```python
from build123d import *

# Parameters (mm, degrees)
F0_W     = 115
F0_H     = 215
F1_DEPTH = 50
F2_W     = 85
F2_H     = 12
F3_DEPTH = 14
F4_R     = 2
F5_DEPTH = 5
F6_R     = 2
F7_DEPTH = 5


with BuildPart() as f1:
    # F0 (on Front) → F1 (new body)
    with BuildSketch(Plane.XZ):
        with Locations((57.5, 107.5)):
            Rectangle(F0_W, F0_H)
    extrude(amount=F1_DEPTH)

    # F2 (on face) → F3 (join)
    with BuildSketch(Plane.XY.offset(215)):
        with Locations((52.5, -36)):
            Rectangle(F2_W, F2_H)
    extrude(amount=F3_DEPTH)

    # F4 (on face) → F5 (cut)
    with BuildSketch(Plane.XZ.offset(50)):
        with Locations((32.5, 182.5)):
            Circle(F4_R)
        with Locations((82.5, 182.5)):
            Circle(F4_R)
        with Locations((82.5, 32.5)):
            Circle(F4_R)
        with Locations((32.5, 32.5)):
            Circle(F4_R)
    extrude(amount=-F5_DEPTH, mode=Mode.SUBTRACT)

    # F6 (on face) → F7 (cut)
    with BuildSketch(Plane(origin=(0, 0, 0), x_dir=(0, -1, 0), z_dir=(-1, 0, 0))):
        with Locations((12.5, 182.5)):
            Circle(F6_R)
        with Locations((37.5, 182.5)):
            Circle(F6_R)
        with Locations((37.5, 32.5)):
            Circle(F6_R)
        with Locations((12.5, 32.5)):
            Circle(F6_R)
    extrude(amount=-F7_DEPTH, mode=Mode.SUBTRACT)


solid = f1.part
```
Geometry check sheet. Reference: the model listing, model coordinates, mm. A direction names the side the tool comes from. Give positions to 0.01 mm unless a question says otherwise; leave off trailing zeros. Write each loop counter-clockwise with the first axis right and the second up, starting at its lowest first coordinate (ties: lowest second). Pieces come first, ordered by that corner, then holes. Notation, with made-up numbers: (-13.5, -38) - (41.5, -38) arc R18 cw to (41.5, -21) - close; hole circle Ø3 at (55, 51.5). An arc over 180 degrees is marked (long way). Use a Markdown table: item, result.
Q1. Section check B-B, the plane y = -23.5. Enter the section's corners in (x, z), then the cut area to 3 significant figures.
Computed:
| item | result |
|---|---|
| outline | (0, 0) - (115, 0) - (115, 215) - (0, 215) - close |
| area | 24,700 mm² |
Q2. Go/stop test with flat-tipped pins: P1, Ø1.2, axis at x = 33, z = 33, coming from the -Y side; P2, Ø7, axis at x = 36, z = 222.5, coming from the -Y side; P3, Ø6, axis at y = -35.5, z = 219.5, coming from the +X side. Record where each tip stops, or that it passes through.
Computed:
| item | result |
|---|---|
| P1 | stops at y = -45 |
| P2 | stops at y = -42 |
| P3 | stops at x = 95 |
Q3. Section check A-A, the plane x = 46. Enter the section's corners in (y, z).
Computed:
| item | result |
|---|---|
| outline | (-50, 0) - (0, 0) - (0, 215) - (-30, 215) - (-30, 229) - (-42, 229) - (-42, 215) - (-50, 215) - close |
Q4. Set-up check for faces 5 (the face through (95, -36, 222)), 6 (the face through (83.423, -47.535, 30.726)), 7 (the face through (2.465, -12.066, 30.548)): record each of +Z, -Z, +X, -X, +Y, -Y from which the full face is reachable in a straight line by a thin tool's end or side.
Computed:
| item | result |
|---|---|
| face 5 | +Z, +X, +Y, -Y |
| face 6 | -Y |
| face 7 | -X |
Q5. Draft check along Z on faces 1 (the face through (32, -45, 183)), 2 (the face through (32, -45, 33)), 3 (the face through (52, -30, 222)), 4 (the face through (57, -25, 0)). Enter one of: pulls with the +Z half, pulls with the -Z half, needs draft (parallel to the pull), parting line crosses it, or undercut.
Computed:
| item | result |
|---|---|
| face 1 | undercut |
| face 2 | undercut |
| face 3 | needs draft |
| face 4 | pulls with the -Z half |
Q6. Thickness scan on L1, parallel to Z at x = 3.5, y = -37.5; L2, parallel to X at y = -47, z = 32; L3, parallel to Z at x = 1, y = -37. Record the ranges inside material, lowest first. Write a range as [from, to].
Computed:
| item | result |
|---|---|
| L1 | z = [0, 30.5], [34.5, 180.5], [184.5, 215] |
| L2 | x = [0, 30.56], [34.44, 80.56], [84.44, 115] |
| L3 | z = [0, 30.56], [34.44, 180.56], [184.44, 215] |
